The listing builds one solid part. Answer for the finished solid, in the listing's coordinates (mm). A direction names the side the tool comes from. Round coordinates to 2 decimals unless told otherwise and drop trailing zeros. Loops run counter-clockwise (first coordinate to the right, second up) from the corner with the lowest first, then second, coordinate; pieces in that order, holes last. Notation, with made-up numbers: (-10.5, 71.5) - (32.5, 71.5) arc R28 cw to (32.5, 103.5) - close; hole circle Ø1 at (-36.75, 19.5). An arc over 180 degrees is marked (long way). One line per item, written item: value.
```python
from build123d import *

# Parameters (mm, degrees)
SKETCH1_R           = 2.125
SKETCH1_R_2         = 1.524
BOSS_EXTRUDE1_DEPTH = 6.92


with BuildPart() as part:
    # Sketch1 → Boss-Extrude1 (new body)
    with BuildSketch(Plane.XY):
        with BuildLine():
            Line((192.041969112, 105.207722008), (192.041969112, 110.207722008))
            Line((192.041969112, 110.207722008), (194.076969112, 110.207722008))
            Line((194.076969112, 110.207722008), (194.076969112, 121.207722008))
            Line((194.076969112, 121.207722008), (170.851969112, 121.207722008))
            Line((170.851969112, 121.207722008), (170.851969112, 125.707722008))
            ThreePointArc((170.851969112, 125.707722008), (170.266182674, 127.12193557), (168.851969112, 127.707722008))
            Line((168.851969112, 127.707722008), (157.851969112, 127.707722008))
            ThreePointArc((157.851969112, 127.707722008), (156.43775555, 127.12193557), (155.851969112, 125.707722008))
            Line((155.851969112, 125.707722008), (155.851969112, 121.207722008))
            Line((155.851969112, 121.207722008), (55.851969112, 121.207722008))
            Line((55.851969112, 121.207722008), (55.851969112, 125.707722008))
            ThreePointArc((55.851969112, 125.707722008), (55.266182674, 127.12193557), (53.851969112, 127.707722008))
            Line((53.851969112, 127.707722008), (42.851969112, 127.707722008))
            ThreePointArc((42.851969112, 127.707722008), (41.43775555, 127.12193557), (40.851969112, 125.707722008))
            Line((40.851969112, 125.707722008), (40.851969112, 121.207722008))
            Line((40.851969112, 121.207722008), (17.626969112, 121.207722008))
            Line((17.626969112, 121.207722008), (17.626969112, 110.207722008))
            Line((17.626969112, 110.207722008), (19.661969112, 110.207722008))
            Line((19.661969112, 110.207722008), (19.661969112, 105.207722008))
            Line((19.661969112, 105.207722008), (17.626969112, 105.207722008))
            Line((17.626969112, 105.207722008), (17.626969112, 100.207722008))
            Line((17.626969112, 100.207722008), (14.076969112, 100.207722008))
            Line((14.076969112, 100.207722008), (14.076969112, 105.207722008))
            Line((14.076969112, 105.207722008), (12.041969112, 105.207722008))
            Line((12.041969112, 105.207722008), (12.041969112, 110.207722008))
            Line((12.041969112, 110.207722008), (14.076969112, 110.207722008))
            Line((14.076969112, 110.207722008), (14.076969112, 121.207722008))
            Line((14.076969112, 121.207722008), (2.851969112, 121.207722008))
            Line((2.851969112, 121.207722008), (2.851969112, 6.207722008))
            Line((2.851969112, 6.207722008), (14.076969112, 6.207722008))
            Line((14.076969112, 6.207722008), (14.076969112, 17.207722008))
            Line((14.076969112, 17.207722008), (12.041969112, 17.207722008))
            Line((12.041969112, 17.207722008), (12.041969112, 22.207722008))
            Line((12.041969112, 22.207722008), (14.076969112, 22.207722008))
            Line((14.076969112, 22.207722008), (14.076969112, 27.207722008))
            Line((14.076969112, 27.207722008), (17.626969112, 27.207722008))
            Line((17.626969112, 27.207722008), (17.626969112, 22.207722008))
            Line((17.626969112, 22.207722008), (19.661969112, 22.207722008))
            Line((19.661969112, 22.207722008), (19.661969112, 17.207722008))
            Line((19.661969112, 17.207722008), (17.626969112, 17.207722008))
            Line((17.626969112, 17.207722008), (17.626969112, 6.207722008))
            Line((17.626969112, 6.207722008), (40.851969112, 6.207722008))
            Line((40.851969112, 6.207722008), (40.851969112, 1.707722008))
            ThreePointArc((40.851969112, 1.707722008), (41.43775555, 0.293508445), (42.851969112, -0.292277992))
            Line((42.851969112, -0.292277992), (53.851969112, -0.292277992))
            ThreePointArc((53.851969112, -0.292277992), (55.266182674, 0.293508445), (55.851969112, 1.707722008))
            Line((55.851969112, 1.707722008), (55.851969112, 6.207722008))
            Line((55.851969112, 6.207722008), (155.851969112, 6.207722008))
            Line((155.851969112, 6.207722008), (155.851969112, 1.707722008))
            ThreePointArc((155.851969112, 1.707722008), (156.43775555, 0.293508445), (157.851969112, -0.292277992))
            Line((157.851969112, -0.292277992), (168.851969112, -0.292277992))
            ThreePointArc((168.851969112, -0.292277992), (170.266182674, 0.293508445), (170.851969112, 1.707722008))
            Line((170.851969112, 1.707722008), (170.851969112, 6.207722008))
            Line((170.851969112, 6.207722008), (194.076969112, 6.207722008))
            Line((194.076969112, 6.207722008), (194.076969112, 17.207722008))
            Line((194.076969112, 17.207722008), (192.041969112, 17.207722008))
            Line((192.041969112, 17.207722008), (192.041969112, 22.207722008))
            Line((192.041969112, 22.207722008), (194.076969112, 22.207722008))
            Line((194.076969112, 22.207722008), (194.076969112, 27.207722008))
            Line((194.076969112, 27.207722008), (197.626969112, 27.207722008))
            Line((197.626969112, 27.207722008), (197.626969112, 22.207722008))
            Line((197.626969112, 22.207722008), (199.661969112, 22.207722008))
            Line((199.661969112, 22.207722008), (199.661969112, 17.207722008))
            Line((199.661969112, 17.207722008), (197.626969112, 17.207722008))
            Line((197.626969112, 17.207722008), (197.626969112, 6.207722008))
            Line((197.626969112, 6.207722008), (208.851969112, 6.207722008))
            Line((208.851969112, 6.207722008), (208.851969112, 121.207722008))
            Line((208.851969112, 121.207722008), (197.626969112, 121.207722008))
            Line((197.626969112, 121.207722008), (197.626969112, 110.207722008))
            Line((197.626969112, 110.207722008), (199.661969112, 110.207722008))
            Line((199.661969112, 110.207722008), (199.661969112, 105.207722008))
            Line((199.661969112, 105.207722008), (197.626969112, 105.207722008))
            Line((197.626969112, 105.207722008), (197.626969112, 100.207722008))
            Line((197.626969112, 100.207722008), (194.076969112, 100.207722008))
            Line((194.076969112, 100.207722008), (194.076969112, 105.207722008))
            Line((194.076969112, 105.207722008), (192.041969112, 105.207722008))
        make_face()
        with Locations((13.851969112, 38.707722008)):
            Circle(SKETCH1_R, mode=Mode.SUBTRACT)
        with Locations((197.851969112, 88.707722008)):
            Circle(SKETCH1_R, mode=Mode.SUBTRACT)
        with Locations((13.851969112, 88.707722008)):
            Circle(SKETCH1_R, mode=Mode.SUBTRACT)
        with Locations((197.851969112, 38.707722008)):
            Circle(SKETCH1_R, mode=Mode.SUBTRACT)
        with Locations((9.851969112, 63.707722008)):
            Circle(SKETCH1_R_2, mode=Mode.SUBTRACT)
        with Locations((201.851969112, 63.707722008)):
            Circle(SKETCH1_R_2, mode=Mode.SUBTRACT)
        with BuildLine():
            Line((19.851969112, 81.093745168), (19.851969112, 46.321698847))
            ThreePointArc((19.851969112, 46.321698847), (20.079852817, 43.716976182), (20.7565798, 41.191396698))
            Line((20.7565798, 41.191396698), (27.455042904, 22.787520574))
            ThreePointArc((27.455042904, 22.787520574), (31.116204748, 18.016201565), (36.851969112, 16.207722008))
            Line((36.851969112, 16.207722008), (174.851969112, 16.207722008))
            ThreePointArc((174.851969112, 16.207722008), (180.587733475, 18.016201565), (184.24889532, 22.787520574))
            Line((184.24889532, 22.787520574), (190.947358424, 41.191396698))
            ThreePointArc((190.947358424, 41.191396698), (191.624085407, 43.716976182), (191.851969112, 46.321698847))
            Line((191.851969112, 46.321698847), (191.851969112, 81.093745168))
            ThreePointArc((191.851969112, 81.093745168), (191.624085407, 83.698467833), (190.947358424, 86.224047318))
            Line((190.947358424, 86.224047318), (184.24889532, 104.627923441))
            ThreePointArc((184.24889532, 104.627923441), (180.587733475, 109.399242451), (174.851969112, 111.207722008))
            Line((174.851969112, 111.207722008), (36.851969112, 111.207722008))
            ThreePointArc((36.851969112, 111.207722008), (31.116204748, 109.399242451), (27.455042904, 104.627923441))
            Line((27.455042904, 104.627923441), (20.7565798, 86.224047318))
            ThreePointArc((20.7565798, 86.224047318), (20.079852817, 83.698467833), (19.851969112, 81.093745168))
        make_face(mode=Mode.SUBTRACT)
    extrude(amount=BOSS_EXTRUDE1_DEPTH)


solid = part.part
```
1) A cutting plane is placed at B-B on y = 108. Give the vertices of the cut face in (x, z).
Final values:
outline: (2.85, 0) - (12.04, 0) - (12.04, 6.92) - (2.85, 6.92) - close; (19.66, 0) - (29.51, 0) - (29.51, 6.92) - (19.66, 6.92) - close; (182.19, 0) - (192.04, 0) - (192.04, 6.92) - (182.19, 6.92) - close; (199.66, 0) - (208.85, 0) - (208.85, 6.92) - (199.66, 6.92) - close
2) For faces 4 (the flat face through (17.627, 12, 3)), 5 (the flat face through (203, 121.208, 3)), 6 (the flat face through (14.077, 103, 3)), determine the directions among +Z, -Z, +X, -X, +Y, -Y from which every point of the face is accessible in a straight line to the end or side of a thin tool.
Final values:
face 4: +Z, -Z, -Y
face 5: +Z, -Z, +X, +Y
face 6: +Z, -Z, +Y
3) A cutting plane is placed at A-A on x = 163.5. Give the vertices of the cut face in (y, z), and give its area (3 significant figures).
Final values:
outline: (-0.29, 0) - (16.21, 0) - (16.21, 6.92) - (-0.29, 6.92) - close; (111.21, 0) - (127.71, 0) - (127.71, 6.92) - (111.21, 6.92) - close
area: 228 mm2
4) A cutting plane is placed at C-C on y = 78. Give the vertices of the cut face in (x, z).
Final values:
outline: (2.85, 0) - (19.85, 0) - (19.85, 6.92) - (2.85, 6.92) - close; (191.85, 0) - (208.85, 0) - (208.85, 6.92) - (191.85, 6.92) - close
5) For a pull along X with two mould halves and no side action, classify faces 1 (the flat face through (40.852, 123, 3)), 2 (the flat face through (8, 6.208, 3)), 3 (the flat face through (107, 121.208, 3)) as released by +X, released by -X, zero draft, split by the parting line, or undercut.
Final values:
face 1: released by -X
face 2: zero draft
face 3: undercut
6) Each of these flat-tipped pins is pushed along its axis until it touches: pin 1 Ø1 at (x, z) = (18.5, 3.5) entering from +Y; pin 2 Ø1.3 at (y, z) = (124, 2.5) entering from -X; pin 3 Ø1.3 at (y, z) = (123, 2.5) entering from +X. Where does it stop, or does it pass through?
Final values:
pin 1: y = 121.21
pin 2: x = 40.85
pin 3: x = 170.85
7) Consider L1, parallel to Y at x = 198, z = 3.75; L2, parallel to X at y = 69, z = 5.75; L3, parallel to X at y = 113.5, z = 0.5. Determine where each line is inside the solid, lowest interval first.
Final values:
L1: 6.21 to 17.21, 22.21 to 36.59, 40.83 to 86.59, 90.83 to 105.21, 110.21 to 121.21
L2: 2.85 to 19.85, 191.85 to 208.85
L3: 2.85 to 14.08, 17.63 to 194.08, 197.63 to 208.85
8) A cutting plane is placed at D-D on z = 3. Give the number of separate pieces and of enclosed holes in the cut face, and give its area (3 significant figures).
Final values:
separate pieces: 1
enclosed holes: 7
area: 7,870 mm2
